Here's how the part is built. I have some questions about the finished solid (model axes, mm). Face numbers are marked on the shaded views. Coordinates: 2 decimals unless noted, no trailing zeros. Write each loop counter-clockwise with the first axis right and the second up, starting at its lowest first coordinate (ties: lowest second). Pieces come first, ordered by that corner, then holes. Notation, with made-up numbers: (11, 3.5) -> (30, 3.5) arc R25 ccw to (30, 34.5) -> close; hole circle Ø5 at (-12.5, -3). An arc over 180 degrees is marked (long way). Use a Markdown table: item, result. Add a question column.
Item 1: Imagine slicing it at A-A, the plane z = -33.5. Write out the boundary of the cut face in (x, y).
Item 2: If we mould it in two halves opening along Z, with no side actions, what happens to the marked faces 1, 2, 3 and 4? For each: pulls with the +Z half, pulls with the -Z half, needs draft (parallel to the pull), parting line crosses it, or undercut.
Item 3: If I drill on line 1 along Z through (x, y) = (45.72, 2.45); line 2 along Z through (x, y) = (45, 4); line 3 along X through (y, z) = (22.5, -10.5), over which ranges is the centre line in solid material (lowest first)? Write a range as from..to.
Item 4: Will these pins go through, and if not, where does the flat tip stop? pin 1 Ø8 at (x, z) = (66, -88) entering from -Y; pin 2 Ø1.1 at (y, z) = (78, -10) entering from +X; pin 3 Ø3 at (x, y) = (38, 12.5) entering from -Z; pin 4 Ø17 at (x, y) = (32.5, 60) entering from +Z.
Item 5: Imagine slicing it at D-D, the plane z = -54.5. Write out the boundary of the cut face in (x, y), and give its area (3 significant figures).
Item 6: Imagine slicing it at B-B, the plane y = 56.5. Write out the boundary of the cut face in (x, z).
```python
from build123d import *

# Parameters (mm, degrees)
SKETCH2_W               = 88.9
SKETCH2_H               = 152.4
BOSS_EXTRUDE1_DEPTH     = 5.9944
CUT_EXTRUDE2_DEPTH      = 177.535840076
CUT_EXTRUDE2_DEPTH_BACK = 177.535840076
SKETCH4_R               = 2.7305
BOSS_EXTRUDE2_DEPTH     = 101.6
FILLET1_R               = 3.81
FILLET2_R               = 2.54
BOSS_EXTRUDE3_DEPTH     = 20.32
FILLET3_R               = 3.81
FILLET6_R               = 3.81
FILLET7_R               = 2.54
CUT_EXTRUDE3_DEPTH      = 204.596488182
CUT_EXTRUDE3_DEPTH_BACK = 204.596488182
SKETCH7_W               = 2.54
SKETCH7_H               = 152.4


with BuildPart() as part:
    # Sketch2 → Boss-Extrude1 (new body)
    with BuildSketch(Plane(origin=(0, 0, 0), x_dir=(1, 0, 0), z_dir=(0, 1, 0))):
        with Locations((44.45, 76.2)):
            Rectangle(SKETCH2_W, SKETCH2_H)
    extrude(amount=BOSS_EXTRUDE1_DEPTH)

    # Sketch4 → Cut-Extrude2 (cut, two sides: drawn at the far end of the back side and taken through both)
    with BuildSketch(Plane(origin=(0, 5.9944, 0), x_dir=(1, 0, 0), z_dir=(0, 1, 0)).offset(-CUT_EXTRUDE2_DEPTH_BACK)):
        with Locations(Location((45.72, 109.871331367, 0), (0, 0, 270))):
            Circle(SKETCH4_R)
        with Locations(Location((45.72, 33.671331367, 0), (0, 0, 270))):
            Circle(SKETCH4_R)
    extrude(amount=CUT_EXTRUDE2_DEPTH + CUT_EXTRUDE2_DEPTH_BACK, mode=Mode.SUBTRACT)

    # Sketch5 → Boss-Extrude2 (add)
    with BuildSketch(Plane(origin=(0, 5.9944, 0), x_dir=(1, 0, 0), z_dir=(0, 1, 0))):
        Polygon((18.796, 15.748), (12.7, 15.748), (12.7, 2.54), (76.2, 2.54), (76.2, 15.748), (70.104, 15.748), (70.104, 13.208), (71.12, 13.208), (71.12, 11.43), (70.104, 11.43), (70.104, 7.62), (18.796, 7.62), (18.796, 11.43), (17.78, 11.43), (17.78, 13.208), (18.796, 13.208), align=None)
    extrude(amount=BOSS_EXTRUDE2_DEPTH)

    # Fillet1
    fillet1_edges = [part.edges().sort_by_distance(p)[0] for p in [
        (12.7, 56.7944, -15.748),
        (12.7, 56.7944, -2.54),
        (76.2, 56.7944, -2.54),
        (76.2, 56.7944, -15.748),
    ]]
    fillet(fillet1_edges, radius=FILLET1_R)

    # Fillet2
    fillet2_edges = [part.edges().sort_by_distance(p)[0] for p in [
        (71.247, 5.9944, -15.748),
        (44.45, 5.9944, -2.54),
        (12.7, 5.9944, -9.144),
        (17.653, 5.9944, -15.748),
        (76.2, 5.9944, -9.144),
        (13.815923164, 5.9944, -3.655923164),
        (13.815923164, 5.9944, -14.632076836),
        (75.084076836, 5.9944, -3.655923164),
        (75.084076836, 5.9944, -14.632076836),
    ]]
    fillet(fillet2_edges, radius=FILLET2_R - 0.0001)  # a hair under: the kernel refuses the full size

    # Sketch6 → Boss-Extrude3 (add, symmetric)
    with BuildSketch(Plane.ZY.offset(-44.45)):
        Polygon((-149.86, 5.9944), (-79.121, 5.9944), (-79.121, 23.1394), (-86.106, 23.1394), (-86.106, 18.0594), (-84.201, 18.0594), (-84.201, 16.1544), (-86.106, 16.1544), (-86.106, 11.0744), (-142.875, 11.0744), (-142.875, 16.1544), (-144.78, 16.1544), (-144.78, 18.0594), (-142.875, 18.0594), (-142.875, 23.1394), (-149.86, 23.1394), align=None)
    extrude(amount=BOSS_EXTRUDE3_DEPTH, both=True)

    # Fillet3
    fillet3_edges = [part.edges().sort_by_distance(p)[0] for p in [
        (44.45, 23.1394, -149.86),
        (44.45, 23.1394, -79.121),
    ]]
    fillet(fillet3_edges, radius=FILLET3_R)

    # Fillet6
    fillet6_edges = [part.edges().sort_by_distance(p)[0] for p in [
        (24.13, 12.6619, -149.86),
        (64.77, 12.6619, -79.121),
        (24.13, 23.1394, -84.5185),
        (24.13, 12.6619, -79.121),
        (64.77, 23.1394, -84.5185),
        (64.77, 12.6619, -149.86),
        (64.77, 23.1394, -144.4625),
        (64.77, 22.023476836, -148.744076836),
        (64.77, 22.023476836, -80.236923164),
        (24.13, 23.1394, -144.4625),
        (24.13, 22.023476836, -148.744076836),
        (24.13, 22.023476836, -80.236923164),
    ]]
    fillet(fillet6_edges, radius=FILLET6_R)

    # Fillet7
    fillet7_edges = [part.edges().sort_by_distance(p)[0] for p in [
        (24.13, 5.9944, -114.4905),
        (64.77, 5.9944, -114.4905),
        (44.45, 5.9944, -79.121),
        (44.45, 5.9944, -149.86),
        (25.245923164, 5.9944, -80.236923164),
        (63.654076836, 5.9944, -80.236923164),
        (63.654076836, 5.9944, -148.744076836),
        (25.245923164, 5.9944, -148.744076836),
    ]]
    fillet(fillet7_edges, radius=FILLET7_R - 0.0001)  # a hair under: the kernel refuses the full size

    # Sketch7 → Cut-Extrude3 (cut, two sides: drawn at the far end of the back side and taken through both)
    with BuildSketch(Plane(origin=(0, 5.9944, 0), x_dir=(1, 0, 0), z_dir=(0, 1, 0)).offset(-CUT_EXTRUDE3_DEPTH_BACK)):
        with Locations((1.27, 76.2)):
            Rectangle(SKETCH7_W, SKETCH7_H)
    extrude(amount=CUT_EXTRUDE3_DEPTH + CUT_EXTRUDE3_DEPTH_BACK, mode=Mode.SUBTRACT)


solid = part.part
```
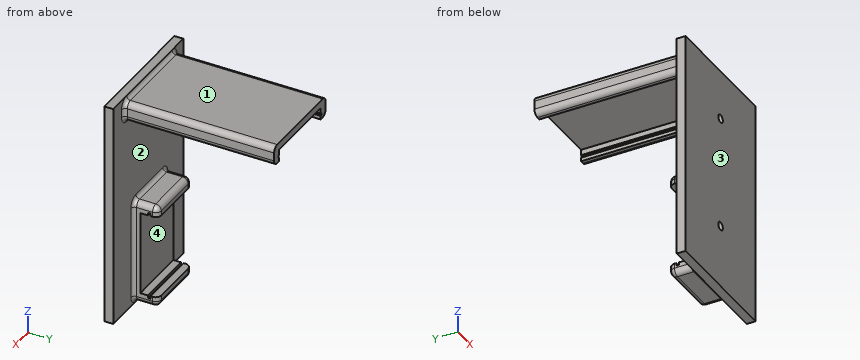
Ans:
| question | item | result |
|---|---|---|
| 1 | outline | (2.54, 0) -> (42.99, 0) -> (42.99, 5.99) -> (2.54, 5.99) -> close; (48.45, 0) -> (88.9, 0) -> (88.9, 5.99) -> (48.45, 5.99) -> close |
| 2 | face 1 | pulls with the +Z half |
| 2 | face 2 | undercut |
| 2 | face 3 | needs draft |
| 2 | face 4 | undercut |
| 3 | line 1 | z = -152.4..-112.6, -107.14..-36.4, -30.94..0 |
| 3 | line 2 | z = -152.4..-112.51, -107.24..-36.31, -31.04..0 |
| 3 | line 3 | x = 12.7..18.8, 70.1..76.2 |
| 4 | pin 1 | stops at y = 0 |
| 4 | pin 2 | stops at x = 76.2 |
| 4 | pin 3 | stops at z = -149.86 |
| 4 | pin 4 | stops at z = -2.54 |
| 5 | outline | (2.54, 0) -> (88.9, 0) -> (88.9, 5.99) -> (2.54, 5.99) -> close |
| 5 | area | 518 mm^2 |
| 6 | outline | (12.7, -11.94) arc R3.81 ccw to (16.51, -15.75) -> (18.8, -15.75) -> (18.8, -13.21) -> (17.78, -13.21) -> (17.78, -11.43) -> (18.8, -11.43) -> (18.8, -7.62) -> (70.1, -7.62) -> (70.1, -11.43) -> (71.12, -11.43) -> (71.12, -13.21) -> (70.1, -13.21) -> (70.1, -15.75) -> (72.39, -15.75) arc R3.81 ccw to (76.2, -11.94) -> (76.2, -6.35) arc R3.81 ccw to (72.39, -2.54) -> (16.51, -2.54) arc R3.81 ccw to (12.7, -6.35) -> close |
